```python
from build123d import *

# Parameters (mm, degrees)
SKETCH_2_R      = 7.1
SKETCH_2_R_2    = 6.1
EXTRUDE_1_DEPTH = 3.2
SKETCH_2_3_R    = 9
SKETCH_2_3_R_2  = 7.1
EXTRUDE_2_DEPTH = 4
EXTRUDE_3_DEPTH = 4
SKETCH_4_W      = 46
SKETCH_4_H      = 30
SKETCH_4_W_2    = 38
SKETCH_4_H_2    = 22
EXTRUDE_4_DEPTH = 4
SKETCH_5_W      = 13
SKETCH_5_H      = 0.8
SKETCH_5_W_2    = 4.5
SKETCH_5_H_2    = 2.4
EXTRUDE_5_DEPTH = 4
FILLET_1_R      = 0.8
FILLET_2_R      = 0.6


with BuildPart() as part:
    # Sketch 2 → Extrude 1 (new body)
    with BuildSketch(Plane.XY):
        Circle(SKETCH_2_R)
        Circle(SKETCH_2_R_2, mode=Mode.SUBTRACT)
    extrude(amount=EXTRUDE_1_DEPTH)

    # Sketch 2_3 → Extrude 2 (add)
    with BuildSketch(Plane.XY):
        Circle(SKETCH_2_3_R)
        Circle(SKETCH_2_3_R_2, mode=Mode.SUBTRACT)
    extrude(amount=EXTRUDE_2_DEPTH)

    # Sketch 3 → Extrude 3 (add)
    with BuildSketch(Plane.XY):
        with BuildLine():
            Line((6, 6.708203932), (6, 9.5))
            Line((6, 9.5), (-6, 9.5))
            Line((-6, 9.5), (-6, 6.708203932))
            ThreePointArc((-6, 6.708203932), (0, 9), (6, 6.708203932))
        make_face()
        with BuildLine():
            Line((-6, -9.5), (6, -9.5))
            Line((6, -9.5), (6, -6.708203932))
            ThreePointArc((6, -6.708203932), (0, -9), (-6, -6.708203932))
            Line((-6, -6.708203932), (-6, -9.5))
        make_face()
    extrude(amount=EXTRUDE_3_DEPTH)



with BuildPart() as body_2:
    # Sketch 4 → Extrude 4 (new body)
    with BuildSketch(Plane.XY):
        Rectangle(SKETCH_4_W, SKETCH_4_H)
        Rectangle(SKETCH_4_W_2, SKETCH_4_H_2, mode=Mode.SUBTRACT)
    extrude(amount=EXTRUDE_4_DEPTH)


with BuildPart() as part_1:
    add(part.part)

    add(body_2.part)  # Extrude 5 merges body 2
    # Sketch 5 → Extrude 5 (add)
    with BuildSketch(Plane.XY):
        with Locations((-12.5, 8)):
            Rectangle(SKETCH_5_W, SKETCH_5_H)
        with Locations((12.5, 8)):
            Rectangle(SKETCH_5_W, SKETCH_5_H)
        with Locations((-12.5, -8)):
            Rectangle(SKETCH_5_W, SKETCH_5_H)
        with Locations((12.5, -8)):
            Rectangle(SKETCH_5_W, SKETCH_5_H)
        with Locations((12.5, 8)):
            Rectangle(SKETCH_5_W_2, SKETCH_5_H_2)
        with Locations((-12.5, 8)):
            Rectangle(SKETCH_5_W_2, SKETCH_5_H_2)
        with Locations((12.5, -8)):
            Rectangle(SKETCH_5_W_2, SKETCH_5_H_2)
        with Locations((-12.5, -8)):
            Rectangle(SKETCH_5_W_2, SKETCH_5_H_2)
    extrude(amount=EXTRUDE_5_DEPTH)

    # Fillet 1
    fillet_1_edges = [part_1.edges().sort_by_distance(p)[0] for p in [
        (19, 7.6, 2),
        (19, -7.6, 2),
        (-19, -7.6, 2),
        (-19, 7.6, 2),
        (-6, 7.6, 2),
        (6, 7.6, 2),
        (6, -7.6, 2),
        (-6, -7.6, 2),
        (-6, -8.4, 2),
        (6, -8.4, 2),
        (6, 8.4, 2),
        (-6, 8.4, 2),
        (-19, 8.4, 2),
        (19, 8.4, 2),
        (-19, -8.4, 2),
        (19, -8.4, 2),
        (-10.25, 7.6, 2),
        (-10.25, 8.4, 2),
        (-14.75, 8.4, 2),
        (-14.75, 7.6, 2),
        (14.75, 7.6, 2),
        (14.75, 8.4, 2),
        (10.25, 8.4, 2),
        (10.25, 7.6, 2),
        (14.75, -8.4, 2),
        (14.75, -7.6, 2),
        (10.25, -7.6, 2),
        (10.25, -8.4, 2),
        (-10.25, -8.4, 2),
        (-10.25, -7.6, 2),
        (-14.75, -7.6, 2),
        (-14.75, -8.4, 2),
    ]]
    fillet(fillet_1_edges, radius=FILLET_1_R - 0.0001)  # a hair under: the kernel refuses the full size

    # Fillet 2
    fillet_2_edges = [part_1.edges().sort_by_distance(p)[0] for p in [
        (-6, -9.5, 2),
        (6, 9.5, 2),
        (6, -9.5, 2),
        (-6, 9.5, 2),
        (6, -6.708203932, 2),
        (-6, 6.708203932, 2),
        (6, 6.708203932, 2),
        (-6, -6.708203932, 2),
    ]]
    fillet(fillet_2_edges, radius=FILLET_2_R)


solid = part_1.part
```
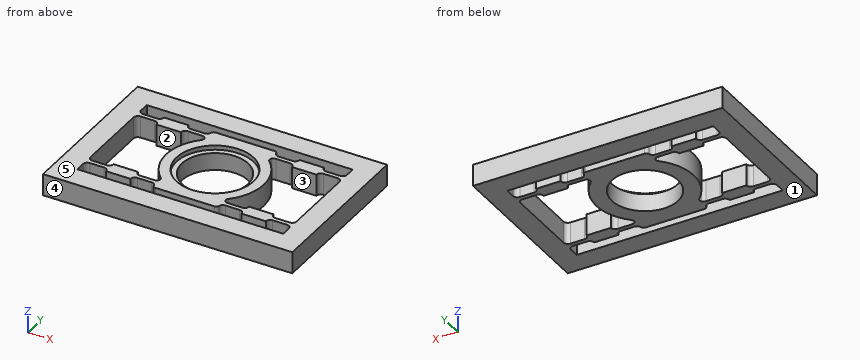
The listing builds one solid part. Answer for the finished solid, in the listing's coordinates (mm). Face numbers are marked on the shaded views. A direction names the side the tool comes from. Coordinates: 2 decimals unless noted, no trailing zeros. Loops run counter-clockwise (first coordinate to the right, second up) from the corner with the lowest first, then second, coordinate; pieces in that order, holes last. Notation, with made-up numbers: (13, 80) -> (49, 80) arc R7 cw to (49, 93) -> close; hole circle Ø2 at (-39.5, 18.5). An arc over 180 degrees is marked (long way). Return JSON: item names as keys, results as strings. Group by question number.
(1) A cutting plane is placed at D-D on z = 2.2. Count the separate pieces of the cut face and the enclosed holes in it, and give its area (4 significant figures).
(2) Determine the mould class of the marked faces 3, 4 and 5 for opening direction Y: released by +Y, released by -Y, zero draft, split by the parting line, or undercut.
(3) A cutting plane is placed at B-B on y = 0. Write down the section's boundary in (x, z), and give its area (3 significant figures).
(4) Find the intervals of material crossed by probe 1 along Y at (x, z) = (0, 2.25); probe 2 along Y at (x, z) = (0, 3.6); probe 3 along X at (y, z) = (-5, 1.65), in increasing order. Write a range as from..to.
(5) A cutting plane is placed at A-A on x = 0. Write down the section's boundary in (y, z), and give its area (3 significant figures).
(6) Which of the six approach directions +Z, -Z, +X, -X, +Y, -Y give full straight-line access (tool end or side, diameter ignored) to the marked faces 1 and 2?
(7) A cutting plane is placed at C-C on x = -16. Write down the section's boundary in (y, z).
The answers:
{
 "1": {"separate pieces": "1", "enclosed holes": "5", "area": "785.5 mm^2"},
 "2": {"face 3": "undercut", "face 4": "released by -Y", "face 5": "zero draft"},
 "3": {"outline": "(-23, 0) -> (-19, 0) -> (-19, 4) -> (-23, 4) -> close; (-9, 0) -> (-6.1, 0) -> (-6.1, 3.2) -> (-7.1, 3.2) -> (-7.1, 4) -> (-9, 4) -> close; (6.1, 0) -> (9, 0) -> (9, 4) -> (7.1, 4) -> (7.1, 3.2) -> (6.1, 3.2) -> close; (19, 0) -> (23, 0) -> (23, 4) -> (19, 4) -> close", "area": "53.6 mm^2"},
 "4": {"probe 1": "y = -15..-11, -9.5..-6.1, 6.1..9.5, 11..15", "probe 2": "y = -15..-11, -9.5..-7.1, 7.1..9.5, 11..15", "probe 3": "x = -23..-19, -7.48..-3.49, 3.49..7.48, 19..23"},
 "5": {"outline": "(-15, 0) -> (-11, 0) -> (-11, 4) -> (-15, 4) -> close; (-9.5, 0) -> (-6.1, 0) -> (-6.1, 3.2) -> (-7.1, 3.2) -> (-7.1, 4) -> (-9.5, 4) -> close; (6.1, 0) -> (9.5, 0) -> (9.5, 4) -> (7.1, 4) -> (7.1, 3.2) -> (6.1, 3.2) -> close; (11, 0) -> (15, 0) -> (15, 4) -> (11, 4) -> close", "area": "57.6 mm^2"},
 "6": {"face 1": "-Z, +X, -X, +Y, -Y", "face 2": "+Z, -Z"},
 "7": {"outline": "(-15, 0) -> (-11, 0) -> (-11, 4) -> (-15, 4) -> close; (-8.4, 0) -> (-7.6, 0) -> (-7.6, 4) -> (-8.4, 4) -> close; (7.6, 0) -> (8.4, 0) -> (8.4, 4) -> (7.6, 4) -> close; (11, 0) -> (15, 0) -> (15, 4) -> (11, 4) -> close"}
}
